Could you check a few things on this drawing? It's one solid part, dimensions in mm from its lowest x, y, z. A direction names the side the tool comes from. Give positions to 0.01 mm unless a question says otherwise; leave off trailing zeros. Order: outer loops, then holes, each group sorted by start corner. A loop starts at its lowest first (then second) coordinate and runs counter-clockwise, first axis right, second up. Notation, with made-up numbers: (68.25, 59.5) - (107.25, 59.5) arc R15 ccw to (107.25, 85.5) - close; hole circle Ø3 at (73.5, 66.25). An arc over 180 degrees is marked (long way). Return JSON: item names as keys, results as strings.
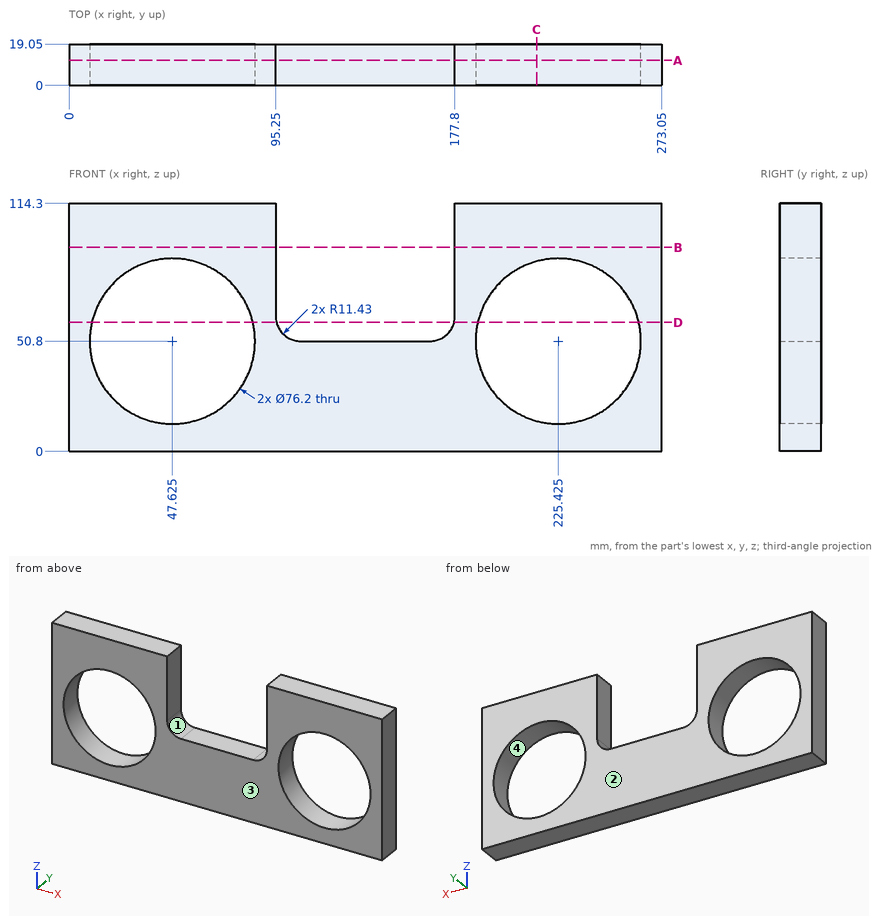
1. If I drill on L1, parallel to X at y = 13.25, z = 29; L2, parallel to X at y = 6, z = 69; L3, parallel to X at y = 17.75, z = 33, over which ranges is the centre line in solid material (lowest first)? Write a range as [from, to].
Checks:
{"L1": "[0, 16.38], [78.87, 194.18], [256.67, 273.05]", "L2": "[0, 14.15], [81.1, 95.25], [177.8, 191.95], [258.9, 273.05]", "L3": "[0, 13.94], [81.31, 191.74], [259.11, 273.05]"}
2. Suppose I cut it at A-A (y = 11.5). List the corners of the cut face in (x, z) for me (3 decimals), plus the area to 3 significant figures.
Checks:
{"outline": "(0, 0) - (273.05, 0) - (273.05, 114.3) - (177.8, 114.3) - (177.8, 62.23) arc R11.43 cw to (166.37, 50.8) - (106.68, 50.8) arc R11.43 cw to (95.25, 62.23) - (95.25, 114.3) - (0, 114.3) - close; hole circle Ø76.2 at (47.625, 50.8); hole circle Ø76.2 at (225.425, 50.8)", "area": "16,900 mm^2"}
3. Thinking about a two-plate mould opening in X: for the marked faces 3 and 4, which applies, +X half, -X half, draft (parallel to the pull), parting line (faces both ways), or undercut?
Checks:
{"face 3": "draft", "face 4": "undercut"}
4. On a 3-axis mill with a long thin cutter (end or side, diameter ignored), from which of +Z, -Z, +X, -X, +Y, -Y can I reach the whole of each face in a straight line? I mean the marked faces 1 and 2. Say none if no direction works.
Checks:
{"face 1": "+Z, +Y, -Y", "face 2": "+Z, -Z, +X, -X, +Y"}
5. For pin 1 Ø5.5 at (x, y) = (125.5, 11.5) entering from +Z, with a flat end and sliding along its axis, tell me the tip position at first contact or that it passes through.
Checks:
{"pin 1": "z = 50.8"}
6. Suppose I cut it at B-B (z = 94). List the corners of the cut face in (x, y) for me, plus the area to 3 significant figures.
Checks:
{"outline": "(0, 0) - (95.25, 0) - (95.25, 19.05) - (0, 19.05) - close; (177.8, 0) - (273.05, 0) - (273.05, 19.05) - (177.8, 19.05) - close", "area": "3,630 mm^2"}
7. Suppose I cut it at D-D (z = 59.5). List the corners of the cut face in (x, y) for me, plus the area to 3 significant figures.
Checks:
{"outline": "(0, 0) - (10.53, 0) - (10.53, 19.05) - (0, 19.05) - close; (84.72, 0) - (95.58, 0) - (95.58, 19.05) - (84.72, 19.05) - close; (177.47, 0) - (188.33, 0) - (188.33, 19.05) - (177.47, 19.05) - close; (262.52, 0) - (273.05, 0) - (273.05, 19.05) - (262.52, 19.05) - close", "area": "815 mm^2"}
8. Suppose I cut it at C-C (x = 215.5). List the corners of the cut face in (y, z) for me.
Checks:
{"outline": "(0, 0) - (19.05, 0) - (19.05, 14.02) - (0, 14.02) - close; (0, 87.58) - (19.05, 87.58) - (19.05, 114.3) - (0, 114.3) - close"}
